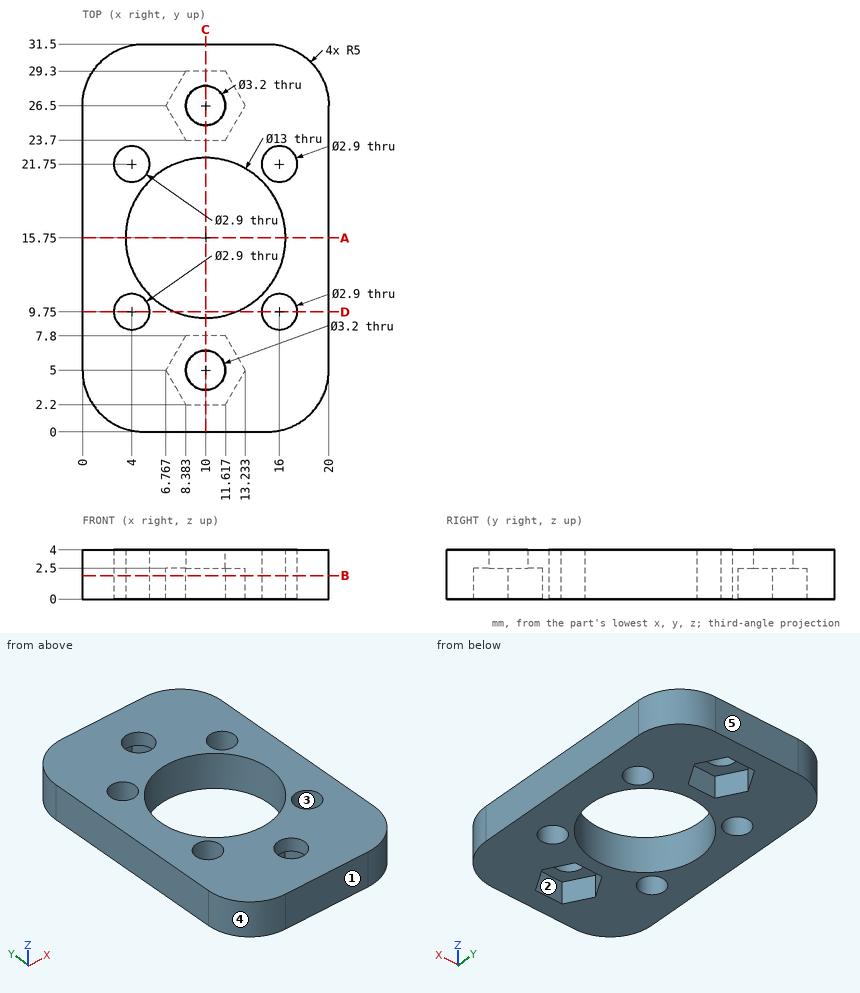
Part print with two shaded views. Sizes in mm from the minimum x, y, z corner. A direction names the side the tool comes from. Give positions to 0.01 mm unless a question says otherwise; leave off trailing zeros. Order: outer loops, then holes, each group sorted by start corner. A loop starts at its lowest first (then second) coordinate and runs counter-clockwise, first axis right, second up.
1) Pin check, flat tips, straight feed: pin 1 (3.5 mm diameter, centred on x = 10, y = 5, fed in from -Z); pin 2 (12 mm diameter, centred on x = 2, y = 12, fed in from -Z); pin 3 (1.7 mm diameter, centred on x = 16, y = 9.75, fed in from +Z). Stop position of each tip, or through.
2) Saw through at B-B, the plane z = 1.9. Write the cut outline in (x, y).
3) Wall check: probe 1 along Y at (x, z) = (10, 1.8); probe 2 along X at (y, z) = (26.5, 3.6); probe 3 along Y at (x, z) = (10, 3.3). Give the ranges that are in metal, low to high.
4) 3-axis set-ups, long thin cutter, end or side, ignore diameter. For the marked faces 1 and 2: which of +Z, -Z, +X, -X, +Y, -Y reach the whole face in a straight line?
5) Saw through at C-C, the plane x = 10. Write the cut outline in (y, z).
6) Mould opens along Y. For the marked faces 3, 4 and 5 say: +Y half, -Y half, draft (parallel to the pull), parting line (faces both ways), or undercut.
7) Saw through at A-A, the plane y = 15.75. Write the cut outline in (x, z), then the cut area to 3 significant figures.
8) Saw through at D-D, the plane y = 9.75. Write the cut outline in (x, z), then the cut area to 3 significant figures.
Computed:
1. pin 1: stops at z = 2.5
1. pin 2: stops at z = 0
1. pin 3: passes through
2. outline: (0, 5) arc R5 ccw to (5, 0) - (15, 0) arc R5 ccw to (20, 5) - (20, 26.5) arc R5 ccw to (15, 31.5) - (5, 31.5) arc R5 ccw to (0, 26.5) - close; hole circle Ø2.9 at (4, 9.75); hole circle Ø2.9 at (4, 21.75); hole circle Ø13 at (10, 15.75); hole (6.77, 5) - (8.38, 2.2) - (11.62, 2.2) - (13.23, 5) - (11.62, 7.8) - (8.38, 7.8) - close; hole (6.77, 26.5) - (8.38, 23.7) - (11.62, 23.7) - (13.23, 26.5) - (11.62, 29.3) - (8.38, 29.3) - close; hole circle Ø2.9 at (16, 9.75); hole circle Ø2.9 at (16, 21.75)
3. probe 1: y = 0 to 2.2, 7.8 to 9.25, 22.25 to 23.7, 29.3 to 31.5
3. probe 2: x = 0 to 8.4, 11.6 to 20
3. probe 3: y = 0 to 3.4, 6.6 to 9.25, 22.25 to 24.9, 28.1 to 31.5
4. face 1: +Z, -Z, +X, -X, -Y
4. face 2: -Z
5. outline: (0, 0) - (2.2, 0) - (2.2, 2.5) - (3.4, 2.5) - (3.4, 4) - (0, 4) - close; (6.6, 2.5) - (7.8, 2.5) - (7.8, 0) - (9.25, 0) - (9.25, 4) - (6.6, 4) - close; (22.25, 0) - (23.7, 0) - (23.7, 2.5) - (24.9, 2.5) - (24.9, 4) - (22.25, 4) - close; (28.1, 2.5) - (29.3, 2.5) - (29.3, 0) - (31.5, 0) - (31.5, 4) - (28.1, 4) - close
6. face 3: undercut
6. face 4: -Y half
6. face 5: +Y half
7. outline: (0, 0) - (3.5, 0) - (3.5, 4) - (0, 4) - close; (16.5, 0) - (20, 0) - (20, 4) - (16.5, 4) - close
7. area: 28.0 mm2
8. outline: (0, 0) - (2.55, 0) - (2.55, 4) - (0, 4) - close; (5.45, 0) - (7.5, 0) - (7.5, 4) - (5.45, 4) - close; (12.5, 0) - (14.55, 0) - (14.55, 4) - (12.5, 4) - close; (17.45, 0) - (20, 0) - (20, 4) - (17.45, 4) - close
8. area: 36.8 mm2
